The figure shows three views and two pictorial views of one solid part (mm, origin at its lowest corner). Answer the questions. A direction names the side the tool comes from. Round coordinates to 2 decimals unless told otherwise and drop trailing zeros. Order: outer loops, then holes, each group sorted by start corner. A loop starts at its lowest first (then second) coordinate and runs counter-clockwise, first axis right, second up. Notation, with made-up numbers: (-16, -38.5) -> (15, -38.5) arc R23 ccw to (15, -6.5) -> close; hole circle Ø6 at (63, 40). An arc over 180 degrees is marked (long way). Return JSON: item names as keys, results as strings. Group by question number.
(1) The part is cut by section B-B (z = 8). Determine the outline of the cut face in (x, y), plus the area to 3 significant figures.
(2) The part is cut by section C-C (y = 10). Determine the outline of the cut face in (x, z), plus the area to 3 significant figures.
(3) Consider line 1 (Y direction, x = 25, z = 5); line 2 (Z direction, x = 39, y = 21.25); line 3 (Y direction, x = 27.5, z = 8.5). Determine where each line is inside the solid, lowest interval first. Write a range as [from, to].
(4) Which of the six approach directions +Z, -Z, +X, -X, +Y, -Y give full straight-line access (tool end or side, diameter ignored) to the marked faces 1, 2 and 3?
(5) Determine the mould class of the marked faces 4, 5 and 6 for opening direction Y: +Y half, -Y half, draft (parallel to the pull), parting line (faces both ways), or undercut.
(6) The part is cut by section A-A (x = 25.4). Determine the outline of the cut face in (y, z), plus the area to 3 significant figures.
(7) Each of these flat-tipped pins is pushed along its axis until it touches: pin 1 (7.5 mm diameter, centred on x = 25.4, y = 12.7, fed in from +Z); pin 2 (7.5 mm diameter, centred on x = 34, y = 17, fed in from +Z). Where does it stop, or does it pass through?
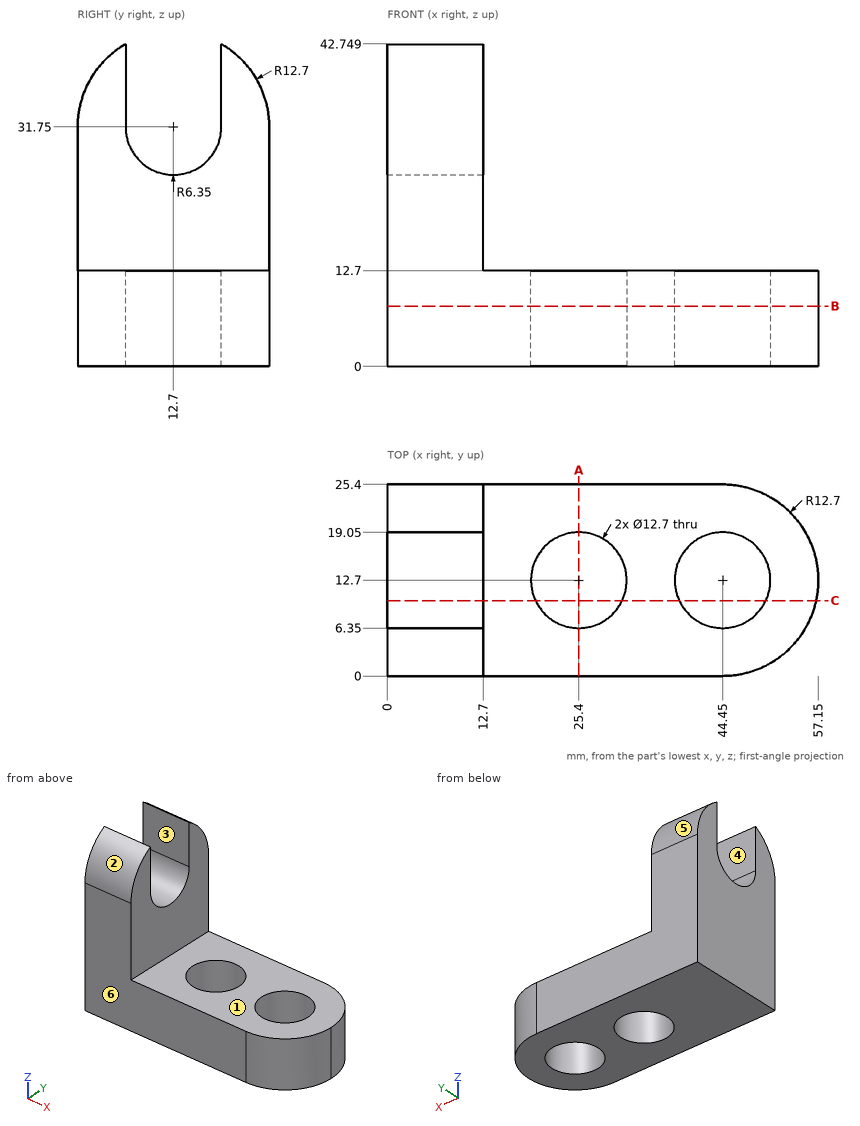
Answer below:
{
 "1": {"outline": "(0, 0) -> (44.45, 0) arc R12.7 ccw to (44.45, 25.4) -> (0, 25.4) -> close; hole circle Ø12.7 at (25.4, 12.7); hole circle Ø12.7 at (44.45, 12.7)", "area": "1,130 mm²"},
 "2": {"outline": "(0, 0) -> (19.65, 0) -> (19.65, 12.7) -> (12.7, 12.7) -> (12.7, 26) -> (0, 26) -> close; (31.15, 0) -> (38.7, 0) -> (38.7, 12.7) -> (31.15, 12.7) -> close; (50.2, 0) -> (56.86, 0) -> (56.86, 12.7) -> (50.2, 12.7) -> close", "area": "599 mm²"},
 "3": {"line 1": "y = [0, 6.36], [19.04, 25.4]", "line 2": "z = [0, 12.7]", "line 3": "y = [0, 6.71], [18.69, 25.4]"},
 "4": {"face 1": "+Z, +X, +Y, -Y", "face 2": "+Z, +X, -X, -Y", "face 3": "+Z, +X, -X"},
 "5": {"face 4": "undercut", "face 5": "+Y half", "face 6": "-Y half"},
 "6": {"outline": "(0, 0) -> (6.35, 0) -> (6.35, 12.7) -> (0, 12.7) -> close; (19.05, 0) -> (25.4, 0) -> (25.4, 12.7) -> (19.05, 12.7) -> close", "area": "161 mm²"},
 "7": {"pin 1": "passes through", "pin 2": "stops at z = 12.7"}
}
